Part model, mm, in its own coordinate system. Face numbers are marked on the shaded views. A direction names the side the tool comes from. Round coordinates to 2 decimals unless told otherwise and drop trailing zeros. Loops run counter-clockwise (first coordinate to the right, second up) from the corner with the lowest first, then second, coordinate; pieces in that order, holes last. Notation, with made-up numbers: M 2,-23.5 L 29,-23.5 A23 cw 29,-11.5 Z; hole C -38,68 d4. An arc over 180 degrees is marked long. Answer as CSV lines item,"result". Start each with the question number.
Item 1: Drop flat-ended pins along their axis: pin 1 Ø3 at (y, z) = (226.5, -11.5) entering from -X; pin 2 Ø5 at (x, y) = (24.5, 172) entering from +Z; pin 3 Ø10 at (x, z) = (-22, -21.5) entering from +Y. Give the stop position or say it passes through.
Item 2: Band-saw the part on C-C (y = 196). Give the cut face in (x, z), and give its area (3 significant figures).
Item 3: Mould opens along Z. For the marked faces 5, 6 and 7 say: pulls with the +Z half, pulls with the -Z half, needs draft (parallel to the pull), parting line crosses it, or undercut.
Item 4: Wall check: line 1 (X direction, y = 27, z = 0); line 2 (Y direction, x = 40, z = -15.5); line 3 (X direction, y = 153, z = 0). Give the ranges that are in metal, low to high.
Item 5: Which spindle directions (+Z, -Z, +X, -X, +Y, -Y) get a long thin tool onto all of the face, cutting with end or side? Do the marked faces 1, 2, 3 and 4. Say none if no direction does.
Item 6: Band-saw the part on D-D (y = 223.5). Give the cut face in (x, z).
```python
from build123d import *

# Parameters (mm, degrees)
SKETCH1_R           = 50
BOSS_EXTRUDE2_DEPTH = 30
SKETCH3_R           = 60
BOSS_EXTRUDE3_DEPTH = 30
SKETCH4_R           = 54
BOSS_EXTRUDE4_DEPTH = 149
SKETCH5_R           = 60
BOSS_EXTRUDE5_DEPTH = 54


with BuildPart() as part:
    # Sketch1 → Boss-Extrude2 (new body)
    with BuildSketch(Plane(origin=(0, 0, 0), x_dir=(1, 0, 0), z_dir=(0, 1, 0))):
        with Locations(Location((0, 0, 0), (0, 0, 270))):
            Circle(SKETCH1_R)
    extrude(amount=BOSS_EXTRUDE2_DEPTH)

    # Sketch3 → Boss-Extrude3 (add)
    with BuildSketch(Plane(origin=(0, 30, 0), x_dir=(1, 0, 0), z_dir=(0, 1, 0))):
        with Locations(Location((0, 0, 0), (0, 0, 270))):
            Circle(SKETCH3_R)
    extrude(amount=BOSS_EXTRUDE3_DEPTH)

    # Sketch4 → Boss-Extrude4 (add)
    with BuildSketch(Plane(origin=(0, 60, 0), x_dir=(1, 0, 0), z_dir=(0, 1, 0))):
        with Locations(Location((0, 0, 0), (0, 0, 270))):
            Circle(SKETCH4_R)
    extrude(amount=BOSS_EXTRUDE4_DEPTH)

    # Sketch5 → Boss-Extrude5 (add)
    with BuildSketch(Plane(origin=(0, 209, 0), x_dir=(1, 0, 0), z_dir=(0, 1, 0))):
        with Locations(Location((0, 0, 0), (0, 0, 270))):
            Circle(SKETCH5_R)
    extrude(amount=BOSS_EXTRUDE5_DEPTH)

    # Sketch7 → Cut-Revolve3 (revolve, cut)
    with BuildSketch(Plane.XY, mode=Mode.PRIVATE) as cut_revolve3_sk:
        Polygon((0, 273.958246316), (0, -7.633446841), (-30, -7.633446841), (-30, 37.558235381), (-48.50368091, 37.558235381), (-48.50368091, 51.558235381), (-37.146978401, 51.558235381), (-37.146978401, 220.582243692), (-48.50368091, 220.582243692), (-48.50368091, 273.958246316), align=None)
    revolve(cut_revolve3_sk.sketch.rotate(Axis((0, 273.958246316, 0), (0, -1, 0)), 270), axis=Axis((0, 273.958246316, 0), (0, -1, 0)), mode=Mode.SUBTRACT)


solid = part.part
```
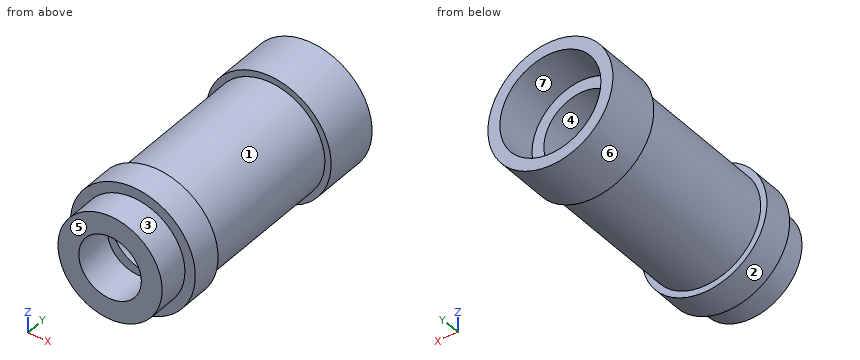
Answer block:
1,pin 1,"stops at x = -59.16"
1,pin 2,"stops at z = 49.32"
1,pin 3,"stops at y = 37.56"
2,outline,"C 0,0 d108; hole C 0,0 d74.29"
2,area,"4,830 mm^2"
3,face 5,"needs draft"
3,face 6,"parting line crosses it"
3,face 7,"undercut"
4,line 1,"x = -50 to -30, 30 to 50"
4,line 2,"y = 0 to 37.56, 51.56 to 220.58"
4,line 3,"x = -54 to -37.15, 37.15 to 54"
5,face 1,"none"
5,face 2,"+Y, -Y"
5,face 3,"-Y"
5,face 4,"+Y"
6,outline,"C 0,0 d120; hole C 0,0 d97.01"
